Source: CAD feature listing. Evaluate the final solid. Frame: model axes, mm. Give positions to 0.01 mm unless a question says otherwise; leave off trailing zeros. Loops run counter-clockwise (first coordinate to the right, second up) from the corner with the lowest first, then second, coordinate; pieces in that order, holes last.
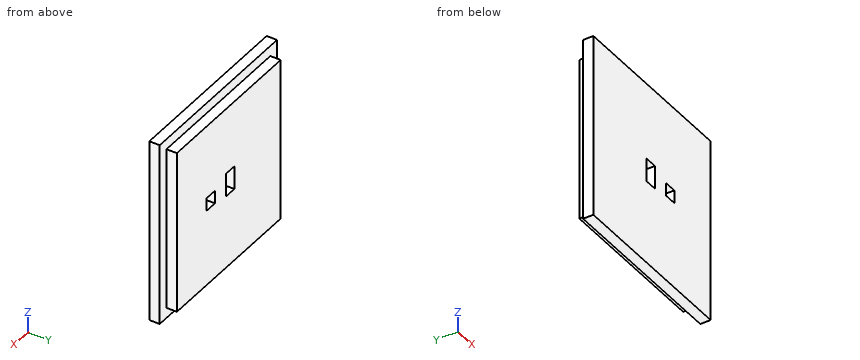
Autodesk Fusion 360 part; units mm, degrees
sketch "Sketch1" plane through (0, 0, 0) normal (0, 1, 0) x (1, 0, 0) in component "Lid"
  line L0 (44.196, 45.085) -> (-44.196, 45.085)
  line L1 (-44.196, 45.085) -> (-44.196, -45.085)
  line L2 (-44.196, -45.085) -> (44.196, -45.085)
  line L3 (44.196, -45.085) -> (44.196, 45.085)
  line L4 (44.196, 45.085) -> (-44.196, -45.085) construction
  line L5 (-44.196, 45.085) -> (44.196, -45.085) construction
  dimension "d1" = 88.392
  dimension "d2" = 90.17
extrude "Extrude1" add sketch "Sketch1" along normal blind 5.08 in component "Lid"
sketch "Sketch3" plane through (0, 5.08, 0) normal (0, 1, 0) x (-1, 0, 0) in component "Lid"
  line L0 (-44.196, 45.085) -> (-44.196, -45.085)
  line L1 (-44.196, -45.085) -> (44.196, -45.085)
  line L2 (44.196, -45.085) -> (44.196, 45.085)
  line L3 (44.196, 45.085) -> (-44.196, 45.085)
  line L4 (-39.116, -40.005) -> (39.116, -40.005)
  line L5 (39.116, -40.005) -> (39.116, 40.005)
  line L6 (39.116, 40.005) -> (-39.116, 40.005)
  line L7 (-39.116, 40.005) -> (-39.116, -40.005)
  line L8 (-39.116, -40.005) -> (39.116, 40.005) construction
  line L9 (39.116, -40.005) -> (-39.116, 40.005) construction
  dimension "d6" = 78.232
  dimension "d7" = 80.01
extrude "Extrude2" add sketch "Sketch3" along normal blind 5.08 contours L4 L5 L6 L7 in component "Lid"
sketch "Sketch6" plane through (0, 0, 0) normal (0, -1, 0) x (1, 0, 0) in component "Lid"
  line L0 (44.196, -45.085) -> (44.196, 45.085)
  line L1 (44.196, 45.085) -> (-44.196, 45.085)
  line L2 (-44.196, 45.085) -> (-44.196, -45.085)
  line L3 (-44.196, -45.085) -> (44.196, -45.085)
  line L4 (2.159, -4.064) -> (-4.191, -4.064)
  line L5 (-4.191, -4.064) -> (-4.191, 7.366)
  line L6 (-4.191, 7.366) -> (2.159, 7.366)
  line L7 (2.159, 7.366) -> (2.159, -4.064)
  line L8 (2.159, -4.064) -> (-4.191, 7.366) construction
  line L9 (-4.191, -4.064) -> (2.159, 7.366) construction
  dimension "d14" = 11.43
  dimension "d15" = 6.35
  dimension "d16" = 1.016
  dimension "d18" = 1.651
extrude "Extrude3" cut sketch "Sketch6" against normal blind 10.16 contours L4 L5 L6 L7 in component "Lid"
sketch "Sketch9" plane through (0, 0, 0) normal (0, 1, 0) x (1, 0, 0) in component "Lid"
  line L0 (16.764, -3.81) -> (10.414, -3.81)
  line L1 (10.414, -3.81) -> (10.414, 2.54)
  line L2 (10.414, 2.54) -> (16.764, 2.54)
  line L3 (16.764, 2.54) -> (16.764, -3.81)
  line L4 (16.764, -3.81) -> (10.414, 2.54) construction
  line L5 (10.414, -3.81) -> (16.764, 2.54) construction
  dimension "d28" = 6.35
  dimension "d29" = 6.35
  dimension "d30" = 0.635
  dimension "d31" = 13.589
extrude "Extrude5" cut sketch "Sketch9" along normal blind 10.16 in component "Lid"
component "Lid" placed x (1, 0, 0) y (0, 1, 0) z (0, 0, 1) at (0, 0, 0)
(1) Section D-D, the plane z = 22. Return the cut outline in (x, y), then the cut area to 3 significant figures.
A:
outline: (-44.2, 0) - (44.2, 0) - (44.2, 5.08) - (39.12, 5.08) - (39.12, 10.16) - (-39.12, 10.16) - (-39.12, 5.08) - (-44.2, 5.08) - close
area: 846 mm2
(2) Ray query, line 1 along X through (y, z) = (1.75, 2); line 2 along Z through (x, y) = (14.5, 6) (3 decimals); line 3 along Z through (x, y) = (-2, 8.5) (3 decimals). Return the intervals inside material, ascending.
A:
line 1: x = -44.2 to -4.19, 2.16 to 10.41, 16.76 to 44.2
line 2: z = -40.005 to -2.54, 3.81 to 40.005
line 3: z = -40.005 to -4.064, 7.366 to 40.005
(3) Section B-B, the plane y = 8.25. Return the cut outline in (x, z) (3 decimals).
A:
outline: (-39.116, -40.005) - (39.116, -40.005) - (39.116, 40.005) - (-39.116, 40.005) - close; hole (-4.191, -4.064) - (2.159, -4.064) - (2.159, 7.366) - (-4.191, 7.366) - close; hole (10.414, -2.54) - (16.764, -2.54) - (16.764, 3.81) - (10.414, 3.81) - close
(4) Section C-C, the plane z = 5.5. Return the cut outline in (x, y).
A:
outline: (-44.2, 0) - (-4.19, 0) - (-4.19, 10.16) - (-39.12, 10.16) - (-39.12, 5.08) - (-44.2, 5.08) - close; (2.16, 0) - (44.2, 0) - (44.2, 5.08) - (39.12, 5.08) - (39.12, 10.16) - (2.16, 10.16) - close
(5) Section A-A, the plane x = 0.5. Return the cut outline in (y, z) (3 decimals), then the cut area to 3 significant figures.
A:
outline: (0, -45.085) - (5.08, -45.085) - (5.08, -40.005) - (10.16, -40.005) - (10.16, -4.064) - (0, -4.064) - close; (0, 7.366) - (10.16, 7.366) - (10.16, 40.005) - (5.08, 40.005) - (5.08, 45.085) - (0, 45.085) - close
area: 748 mm2
(6) First-contact query: pin 1 (1.5 mm diameter, centred on x = -8, y = 8, fed in from +Z) (3 decimals); pin 2 (5.5 mm diameter, centred on x = -2.5, y = 6.5, fed in from -Z) (3 decimals); pin 3 (4 mm diameter, centred on y = 7.5, z = 16.5, fed in from -X); pin 4 (1.9 mm diameter, centred on y = 6.5, z = 1, fed in from +X). Flat tips, straight axial feed; report the tip coordinate or a pass-through.
A:
pin 1: stops at z = 40.005
pin 2: stops at z = -45.085
pin 3: stops at x = -39.12
pin 4: stops at x = 39.12
